```python
from build123d import *

# Parameters (mm, degrees)
SKETCH1_R           = 15
BOSS_EXTRUDE1_DEPTH = 15


with BuildPart() as part:
    # Sketch1 → Boss-Extrude1 (new body)
    with BuildSketch(Plane(origin=(0, 0, 0), x_dir=(1, 0, 0), z_dir=(0, 1, 0))):
        Polygon((30, 0), (15, 25.980762114), (-15, 25.980762114), (-30, 0), (-15, -25.980762114), (15, -25.980762114), align=None)
        with Locations(Location((0, 0, 0), (0, 0, 270))):
            Circle(SKETCH1_R, mode=Mode.SUBTRACT)
    extrude(amount=BOSS_EXTRUDE1_DEPTH)

    # Sketch3 → Cut-Revolve1 (revolve, cut)
    with BuildSketch(Plane.XY, mode=Mode.PRIVATE) as cut_revolve1_sk:
        Polygon((-30, 15), (-30, 10.235882569), (-23.813738417, 15), align=None)
    revolve(cut_revolve1_sk.sketch.rotate(Axis((0, 0, 0), (0, 1, 0)), 270), axis=Axis((0, 0, 0), (0, 1, 0)), mode=Mode.SUBTRACT)


solid = part.part
```
CAD build for the part. Positions are in the model's coordinates, mm. Round coordinates to 2 decimals unless told otherwise and drop trailing zeros. Loops run counter-clockwise (first coordinate to the right, second up) from the corner with the lowest first, then second, coordinate; pieces in that order, holes last. Notation, with made-up numbers: (-28, -22.75) - (-19, -22.75) arc R17 ccw to (-19, -14.75) - close; hole circle Ø9 at (28.5, -21). An arc over 180 degrees is marked (long way). Return JSON: item names as keys, results as strings. Group by question number.
Q1. Band-saw the part on B-B on y = 9.25. Give the cut face in (x, z), plus the area to 3 significant figures.
Q2. Band-saw the part on A-A on x = 0. Give the cut face in (y, z), plus the area to 3 significant figures.
Q3. Flat gauge pins, fed straight in: pin 1 Ø3 at (y, z) = (3, -11.5) entering from -X; pin 2 Ø6 at (y, z) = (13.5, 5.5) entering from -X; pin 3 Ø8 at (y, z) = (8, -20.5) entering from -X; pin 4 Ø1 at (x, z) = (-1, 13.5) entering from +Y. Where does each tip first touch, or does it go through?
Q4. Drill centre lines: line 1 along X through (y, z) = (9.5, 0); line 2 along X through (y, z) = (11, 0); line 3 along Z through (x, y) = (9.5, 10.75). Where is each one in solid material? Low to high. Write a range as [from, to].
Q5. Two-plate mould, pull along Z, no slides. Class faces 1 (the face through (0.66, 7.395, -14.985)), 2 (the face through (0, 7, 25.981)), 3 (the face through (0, 15, 16)): +Z half, -Z half, draft (parallel to the pull), parting line (faces both ways), or undercut.
Solutions:
{
 "1": {"outline": "(-30, 0) - (-15, -25.98) - (15, -25.98) - (30, 0) - (15, 25.98) - (-15, 25.98) - close; hole circle Ø30 at (0, 0)", "area": "1,630 mm^2"},
 "2": {"outline": "(0, -25.98) - (13.33, -25.98) - (15, -23.81) - (15, -15) - (0, -15) - close; (0, 15) - (15, 15) - (15, 23.81) - (13.33, 25.98) - (0, 25.98) - close", "area": "326 mm^2"},
 "3": {"pin 1": "stops at x = -24.23", "pin 2": "stops at x = -28.13", "pin 3": "stops at x = -20.47", "pin 4": "passes through"},
 "4": {"line 1": "x = [-30, -15], [15, 30]", "line 2": "x = [-29.01, -15], [15, 29.01]", "line 3": "z = [-25.98, -11.61], [11.61, 25.98]"},
 "5": {"face 1": "undercut", "face 2": "+Z half", "face 3": "draft"}
}
